from build123d import *

# Parameters (mm, degrees)
CROQUIS1_R              = 2.4500000000000015
SALIENTE_EXTRUIR1_DEPTH = 2
SALIENTE_EXTRUIR2_DEPTH = 5
CROQUIS3_R              = 1.5499999999999992
CORTAR_EXTRUIR1_DEPTH   = 26.03996805109803
CROQUIS4_R              = 5
CORTAR_EXTRUIR2_DEPTH   = 5
CHAFL_N1_SIZE           = 0.5
CHAFL_N2_SIZE           = 0.5


with BuildPart() as part:
    # Croquis1 → Saliente-Extruir1 (new body)
    with BuildSketch(Plane.XY):
        with BuildLine():
            ThreePointArc((-10.049999999999738, -12.5), (-10.76758838609276, -10.767588386092894), (-12.499999999999918, -10.049999999999999))
            Line((-12.499999999999996, -10.049999999999997), (-12.499999999999996, -12.5))
            Line((-12.499999999999996, -12.5), (-10.049999999999738, -12.5))
        make_face()
        with BuildLine():
            Line((-12.499999999999996, -12.5), (-12.499999999999996, -10.049999999999997))
            ThreePointArc((-12.499999999999918, -10.049999999999999), (-14.232411613906718, -14.232411613907106), (-10.049999999999738, -12.5))
            Line((-10.049999999999738, -12.5), (-12.499999999999996, -12.5))
        make_face()
        with BuildLine():
            ThreePointArc((14.950000000000262, -12.5), (14.23241161390724, -10.767588386092894), (12.500000000000082, -10.049999999999999))
            Line((12.500000000000004, -10.05), (12.500000000000004, -12.499999999999996))
            Line((12.500000000000004, -12.499999999999996), (10.05000000000026, -12.499999999999996))
            ThreePointArc((10.05000000000026, -12.5), (12.500000000000261, -14.950000000000001), (14.950000000000262, -12.5))
        make_face()
        with BuildLine():
            Line((12.500000000000004, -12.499999999999996), (12.500000000000004, -10.05))
            ThreePointArc((12.500000000000082, -10.049999999999999), (10.767588386093156, -10.76758838609302), (10.05000000000026, -12.5))
            Line((10.05000000000026, -12.499999999999996), (12.500000000000004, -12.499999999999996))
        make_face()
        with BuildLine():
            ThreePointArc((-12.499999999999922, 10.049999999999999), (-10.76758838609293, 10.767588386092985), (-10.049999999999999, 12.5))
            Line((-10.049999999999997, 12.5), (-12.5, 12.5))
            Line((-12.5, 12.5), (-12.5, 10.049999999999999))
        make_face()
        with BuildLine():
            Line((-12.5, 12.5), (-10.049999999999997, 12.5))
            ThreePointArc((-10.049999999999999, 12.5), (-14.23241161390707, 14.232411613907015), (-12.499999999999922, 10.049999999999999))
            Line((-12.5, 10.049999999999999), (-12.5, 12.5))
        make_face()
        with Locations((12.5, 12.5)):
            Circle(CROQUIS1_R)
    extrude(amount=SALIENTE_EXTRUIR1_DEPTH)

    # Croquis2 → Saliente-Extruir2 (add)
    with BuildSketch(Plane.XY.offset(2)):
        with BuildLine():
            ThreePointArc((-7.999999999999958, 12.499999999999764), (-15.68198051533941, 15.681980515339577), (-12.5, 8))
            ThreePointArc((-12.5, 8), (-9.186291501015104, 5.367e-14), (-12.499999999999739, -8))
            ThreePointArc((-12.499999999999739, -8), (-15.681980515339163, -15.681980515339504), (-7.999999999999414, -12.499999999999883))
            ThreePointArc((-7.999999999999414, -12.499999999999883), (3.2112e-13, -9.18629150101557), (8.000000000000586, -12.499999999999618))
            ThreePointArc((8.000000000000586, -12.499999999999618), (15.681980515339447, -15.681980515339283), (12.500000000000016, -8.000000000000036))
            ThreePointArc((12.500000000000016, -8.000000000000036), (9.186291501015239, -2.647e-14), (12.50000000000002, 7.999999999999989))
            ThreePointArc((12.50000000000002, 7.999999999999989), (15.681980515339454, 15.68198051533949), (8.000000000000043, 12.49999999999997))
            ThreePointArc((8.000000000000043, 12.49999999999997), (8.613e-14, 9.1862915010151), (-7.999999999999958, 12.499999999999764))
        make_face()
    extrude(amount=SALIENTE_EXTRUIR2_DEPTH)

    # Croquis3 → Cortar-Extruir1 (cut, through all)
    with BuildSketch(Plane(origin=(0, 0, 0), x_dir=(-1, 0, 0), z_dir=(0, 0, -1))):
        with Locations((-12.500000000000261, -12.5)):
            Circle(CROQUIS3_R)
        with Locations((12.49999999999974, -12.5)):
            Circle(CROQUIS3_R)
        with Locations((12.499999999999654, 12.5)):
            Circle(CROQUIS3_R)
        with Locations((-12.500000000000348, 12.5)):
            Circle(CROQUIS3_R)
    extrude(amount=-CORTAR_EXTRUIR1_DEPTH, mode=Mode.SUBTRACT)

    # Croquis4 → Cortar-Extruir2 (cut)
    with BuildSketch(Plane.XY.offset(7)):
        Circle(CROQUIS4_R)
    extrude(amount=-CORTAR_EXTRUIR2_DEPTH, mode=Mode.SUBTRACT)

    # Chaflán1
    chafl_n1_edges = [part.edges().sort_by_distance(p)[0] for p in [
        (10.050000000000264, -12.5, 0),
        (-14.949999999999736, -12.5, 0),
        (-12.500000000000078, 14.950000000000001, 0),
        (10.049999999999999, 12.5, 0),
    ]]
    chamfer(chafl_n1_edges, length=CHAFL_N1_SIZE)

    # Chaflán2
    chafl_n2_edges = [part.edges().sort_by_distance(p)[0] for p in [
        (-15.681980515339374, 15.68198051533961, 2),
    ]]
    chamfer(chafl_n2_edges, length=CHAFL_N2_SIZE)
    chafl_n2_2_edges = [part.edges().sort_by_distance(p)[0] for p in [
        (8.438e-14, 9.186291501015104, 2),
    ]]
    chamfer(chafl_n2_2_edges, length=CHAFL_N2_SIZE)
    chafl_n2_3_edges = [part.edges().sort_by_distance(p)[0] for p in [
        (-9.186291501015104, 5.44e-14, 2),
    ]]
    chamfer(chafl_n2_3_edges, length=CHAFL_N2_SIZE)
    chafl_n2_4_edges = [part.edges().sort_by_distance(p)[0] for p in [
        (15.681980515339504, 15.681980515339442, 2),
    ]]
    chamfer(chafl_n2_4_edges, length=CHAFL_N2_SIZE - 0.0001)  # a hair under: the kernel refuses the full size
    chafl_n2_5_edges = [part.edges().sort_by_distance(p)[0] for p in [
        (-15.681980515338884, -15.68198051533978, 2),
    ]]
    chamfer(chafl_n2_5_edges, length=CHAFL_N2_SIZE)
    chafl_n2_6_edges = [part.edges().sort_by_distance(p)[0] for p in [
        (9.186291501015239, -2.132e-14, 2),
    ]]
    chamfer(chafl_n2_6_edges, length=CHAFL_N2_SIZE - 0.0001)  # a hair under: the kernel refuses the full size
    chafl_n2_7_edges = [part.edges().sort_by_distance(p)[0] for p in [
        (5.318e-13, -9.18629150101557, 2),
    ]]
    chamfer(chafl_n2_7_edges, length=CHAFL_N2_SIZE)
    chafl_n2_8_edges = [part.edges().sort_by_distance(p)[0] for p in [
        (15.681980515339694, -15.681980515339037, 2),
    ]]
    chamfer(chafl_n2_8_edges, length=CHAFL_N2_SIZE - 0.0004)  # a hair under: the kernel refuses the full size
    chafl_n2_9_edges = [part.edges().sort_by_distance(p)[0] for p in [
        (-5, 6.1e-16, 2),
    ]]
    chamfer(chafl_n2_9_edges, length=CHAFL_N2_SIZE)


solid = part.part
Geometry check sheet. Reference: the model listing, model coordinates, mm. A direction names the side the tool comes from. Give positions to 0.01 mm unless a question says otherwise; leave off trailing zeros. Loops run counter-clockwise (first coordinate to the right, second up) from the corner with the lowest first, then second, coordinate; pieces in that order, holes last.
(1) Set-up check for faces 4 (the cylindrical face through (-1.08, -4.88, 4.78)), 5 (the cylindrical face through (-14.948, 12.608, 1.24)): record each of +Z, -Z, +X, -X, +Y, -Y from which the full face is reachable in a straight line by a thin tool's end or side.
From the geometry:
face 4: +Z, -Z
face 5: -Z
(2) Thickness scan on L1, parallel to Z at x = 8.5, y = 7.5; L2, parallel to X at y = -2, z = 3; L3, parallel to Y at x = 3, z = 5.5. Record the ranges inside material, lowest first.
From the geometry:
L1: z = 2 to 7
L2: x = -9.36 to -4.58, 4.58 to 9.36
L3: y = -9.59 to -4, 4 to 9.59
(3) Section check A-A on y = 0. Record the cut outline in (x, z), then the cut area to 3 significant figures.
From the geometry:
outline: (-9.19, 2.5) - (-8.69, 2) - (-5.5, 2) - (-5, 2.5) - (-5, 7) - (-9.19, 7) - close; (5, 2.5) - (5.5, 2) - (8.69, 2) - (9.19, 2.5) - (9.19, 7) - (5, 7) - close
area: 41.4 mm2
(4) Depth check by flat-ended pin: pin 1 Ø4 at (y, z) = (7.5, 2) entering from -X; pin 2 Ø4 at (y, z) = (5, 2.5) entering from +X; pin 3 Ø2.5 at (x, y) = (-12.5, 12.5) entering from -Z; pin 4 Ø13 at (x, y) = (0, 0) entering from -Z. Enter the tip coordinate at first touch or a pass-through.
From the geometry:
pin 1: stops at x = -15.8
pin 2: stops at x = 11.61
pin 3: passes through
pin 4: stops at z = 2
(5) Release check for a two-part mould opening along Y. For faces 1 (the cylindrical face through (0.124, 9.187, 4.719)), 2 (the conical face through (0.129, -9.052, 2.365)), 3 (the conical face through (15.526, -15.329, 2.142)) record: released by +Y, released by -Y, zero draft, split by the parting line, or undercut.
From the geometry:
face 1: released by +Y
face 2: released by -Y
face 3: undercut
